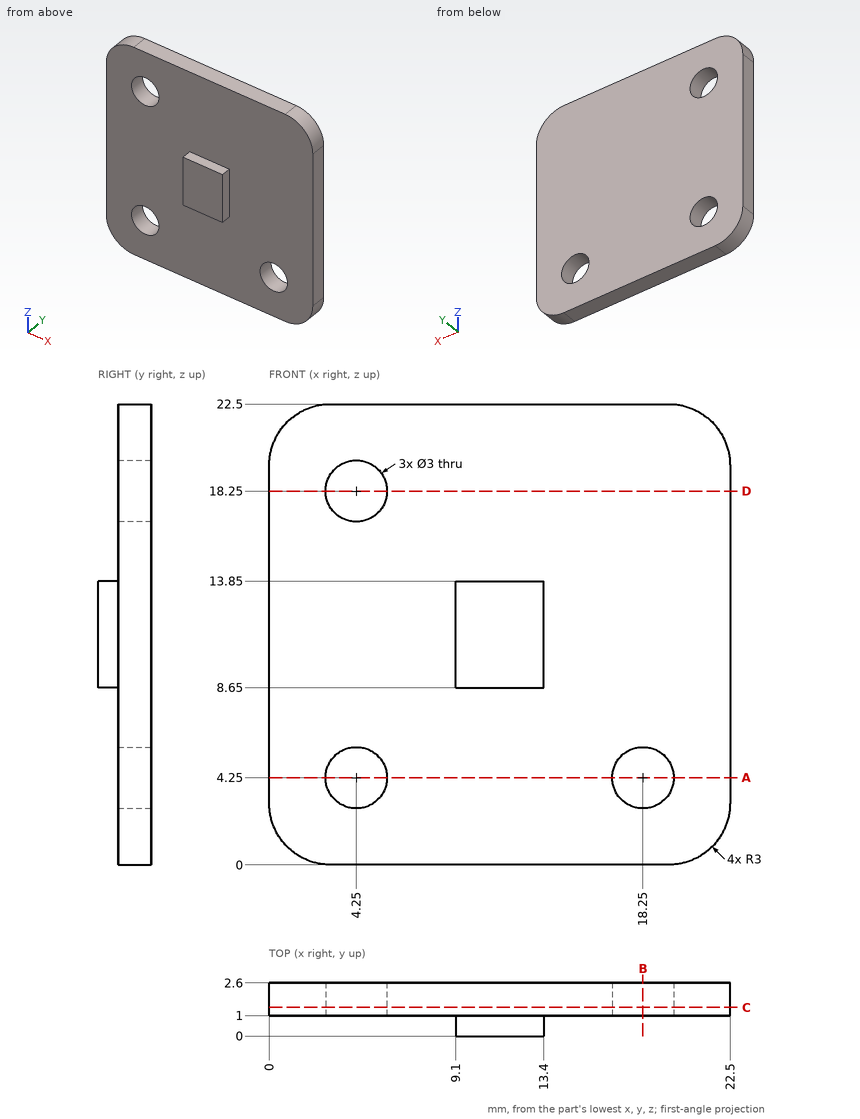
Could you check a few things on this drawing? It's one solid part, dimensions in mm from its lowest x, y, z. Give positions to 0.01 mm unless a question says otherwise; leave off trailing zeros. Loops run counter-clockwise (first coordinate to the right, second up) from the corner with the lowest first, then second, coordinate; pieces in that order, holes last. Notation, with made-up numbers: (12.25, 25) -> (24.25, 25) arc R35 ccw to (24.25, 60) -> close; hole circle Ø5 at (79.25, 9). An arc over 180 degrees is marked (long way). Answer as CSV lines item,"result". Start each with the question number.
(1) If we section it at A-A on z = 4.25: Write out the boundary of the cut face in (x, y), then the cut area to 3 significant figures.
(2) I'm going to push flat-ended pins straight in: pin 1 Ø3.5 at (x, z) = (18.25, 4.25) entering from -Y; pin 2 Ø0.8 at (y, z) = (0.5, 10) entering from -X. Where does each tip first touch, or does it pass through?
(3) I need wall thicknesses on probe 1 along X at (y, z) = (2.35, 4.25); probe 2 along X at (y, z) = (2.1, 18.25); probe 3 along Y at (x, z) = (20, 17.75). Which ranges of each line are inside material? Lowest first, please.
(4) If we section it at C-C on y = 1.4: Write out the boundary of the cut face in (x, z), then the cut area to 3 significant figures.
(5) If we section it at D-D on z = 18.25: Write out the boundary of the cut face in (x, y).
(6) If we section it at B-B on x = 18.25: Write out the boundary of the cut face in (y, z).
Computed:
1,outline,"(0, 1) -> (2.75, 1) -> (2.75, 2.6) -> (0, 2.6) -> close; (5.75, 1) -> (16.75, 1) -> (16.75, 2.6) -> (5.75, 2.6) -> close; (19.75, 1) -> (22.5, 1) -> (22.5, 2.6) -> (19.75, 2.6) -> close"
1,area,"26.4 mm2"
2,pin 1,"stops at y = 1"
2,pin 2,"stops at x = 9.1"
3,probe 1,"x = 0 to 2.75, 5.75 to 16.75, 19.75 to 22.5"
3,probe 2,"x = 0 to 2.75, 5.75 to 22.5"
3,probe 3,"y = 1 to 2.6"
4,outline,"(0, 3) arc R3 ccw to (3, 0) -> (19.5, 0) arc R3 ccw to (22.5, 3) -> (22.5, 19.5) arc R3 ccw to (19.5, 22.5) -> (3, 22.5) arc R3 ccw to (0, 19.5) -> close; hole circle Ø3 at (4.25, 4.25); hole circle Ø3 at (4.25, 18.25); hole circle Ø3 at (18.25, 4.25)"
4,area,"477 mm2"
5,outline,"(0, 1) -> (2.75, 1) -> (2.75, 2.6) -> (0, 2.6) -> close; (5.75, 1) -> (22.5, 1) -> (22.5, 2.6) -> (5.75, 2.6) -> close"
6,outline,"(1, 0) -> (2.6, 0) -> (2.6, 2.75) -> (1, 2.75) -> close; (1, 5.75) -> (2.6, 5.75) -> (2.6, 22.5) -> (1, 22.5) -> close"
